```python
from build123d import *

# Parameters (mm, degrees)
BOSS_EXTRUDE1_DEPTH = 6.1
CUT_EXTRUDE1_DEPTH  = 1


with BuildPart() as part:
    # Sketch1 → Boss-Extrude1 (new body)
    with BuildSketch(Plane(origin=(0, 0, 0), x_dir=(1, 0, 0), z_dir=(0, 1, 0))):
        with BuildLine():
            ThreePointArc((-2.603734293, 13.735096717), (-4.043681259, 12.445171239), (-5.966821997, 12.642363282))
            Line((-5.966821997, 12.642363282), (-6.843279813, 13.183422247))
            Line((-6.843279813, 13.183422247), (-7.052164592, 13.353548445))
            Line((-7.052164592, 13.353548445), (-7.399861002, 13.637560961))
            Line((-7.399861002, 13.637560961), (-7.793732744, 13.973879308))
            Line((-7.793732744, 13.973879308), (-8.226942264, 14.264456075))
            Line((-8.226942264, 14.264456075), (-9.020650473, 14.599698524))
            Line((-9.020650473, 14.599698524), (-9.172029908, 14.639881345))
            Line((-9.172029908, 14.639881345), (-11.091125587, 13.245576719))
            Line((-11.091125587, 13.245576719), (-11.051137643, 12.366770586))
            Line((-11.051137643, 12.366770586), (-10.799290258, 11.512249619))
            Line((-10.799290258, 11.512249619), (-10.485832024, 10.75420757))
            Line((-10.485832024, 10.75420757), (-10.259959226, 9.993083115))
            Line((-10.259959226, 9.993083115), (-10.179752581, 9.581490045))
            ThreePointArc((-10.179752581, 9.581490045), (-10.586494975, 7.691538822), (-12.258255089, 6.720676771))
            Line((-12.258255089, 6.720676771), (-13.285350838, 6.643233691))
            Line((-13.285350838, 6.643233691), (-13.554339843, 6.658089283))
            Line((-13.554339843, 6.658089283), (-14.002570517, 6.683489414))
            Line((-14.002570517, 6.683489414), (-14.518902414, 6.72406467))
            Line((-14.518902414, 6.72406467), (-15.040173016, 6.704512046))
            Line((-15.040173016, 6.704512046), (-15.879347013, 6.509198904))
            Line((-15.879347013, 6.509198904), (-16.025434419, 6.452728891))
            Line((-16.025434419, 6.452728891), (-16.75846374, 4.196696614))
            Line((-16.75846374, 4.196696614), (-16.20956353, 3.509231842))
            Line((-16.20956353, 3.509231842), (-15.503539893, 2.965942036))
            Line((-15.503539893, 2.965942036), (-14.804380918, 2.536919263))
            Line((-14.804380918, 2.536919263), (-14.174268255, 2.053921344))
            Line((-14.174268255, 2.053921344), (-13.86745138, 1.768079839))
            ThreePointArc((-13.86745138, 1.768079839), (-13.085627432, 0), (-13.86745138, -1.768079839))
            Line((-13.86745138, -1.768079839), (-14.652869395, -2.434444341))
            Line((-14.652869395, -2.434444341), (-14.87921797, -2.580533684))
            Line((-14.87921797, -2.580533684), (-15.256774024, -2.823447927))
            Line((-15.256774024, -2.823447927), (-15.698344841, -3.094114129))
            Line((-15.698344841, -3.094114129), (-16.108568873, -3.416327706))
            Line((-16.108568873, -3.416327706), (-16.672672713, -4.067593457))
            Line((-16.672672713, -4.067593457), (-16.757667666, -4.19914668))
            Line((-16.757667666, -4.19914668), (-16.024638344, -6.455178957))
            Line((-16.024638344, -6.455178957), (-15.176487091, -6.688714191))
            Line((-15.176487091, -6.688714191), (-14.285964235, -6.713254596))
            Line((-14.285964235, -6.713254596), (-13.468159483, -6.649385976))
            Line((-13.468159483, -6.649385976), (-12.674488577, -6.66976857))
            Line((-12.674488577, -6.66976857), (-12.258255089, -6.720676771))
            ThreePointArc((-12.258255089, -6.720676771), (-10.586494975, -7.691538822), (-10.179752581, -9.581490045))
            Line((-10.179752581, -9.581490045), (-10.423489876, -10.582247377))
            Line((-10.423489876, -10.582247377), (-10.520740558, -10.833480493))
            Line((-10.520740558, -10.833480493), (-10.683408413, -11.251924125))
            Line((-10.683408413, -11.251924125), (-10.881553106, -11.730446496))
            Line((-10.881553106, -11.730446496), (-11.02403893, -12.232246392))
            Line((-11.02403893, -12.232246392), (-11.09760412, -13.09070337))
            Line((-11.09760412, -13.09070337), (-11.089041437, -13.247090943))
            Line((-11.089041437, -13.247090943), (-9.169945757, -14.641395569))
            Line((-9.169945757, -14.641395569), (-8.346508413, -14.331798745))
            Line((-8.346508413, -14.331798745), (-7.611635801, -13.828216148))
            Line((-7.611635801, -13.828216148), (-6.987558891, -13.295851776))
            Line((-6.987558891, -13.295851776), (-6.333485052, -12.845833588))
            Line((-6.333485052, -12.845833588), (-5.966821997, -12.642363282))
            ThreePointArc((-5.966821997, -12.642363282), (-4.043681259, -12.445171239), (-2.603734293, -13.735096717))
            Line((-2.603734293, -13.735096717), (-2.212691506, -14.687991594))
            Line((-2.212691506, -14.687991594), (-2.14369784, -14.94840597))
            Line((-2.14369784, -14.94840597), (-2.029343904, -15.382547746))
            Line((-2.029343904, -15.382547746), (-1.908377935, -15.886147005))
            Line((-1.908377935, -15.886147005), (-1.72870081, -16.375862714))
            Line((-1.72870081, -16.375862714), (-1.283627947, -17.113609532))
            Line((-1.283627947, -17.113609532), (-1.184778282, -17.235096718))
            Line((-1.184778282, -17.235096718), (1.187354434, -17.235096718))
            Line((1.187354434, -17.235096718), (1.671552791, -16.500623298))
            Line((1.671552791, -16.500623298), (1.970078799, -15.661269135))
            Line((1.970078799, -15.661269135), (2.162051698, -14.863754107))
            Line((2.162051698, -14.863754107), (2.426694495, -14.115226788))
            Line((2.426694495, -14.115226788), (2.603734293, -13.735096717))
            ThreePointArc((2.603734293, -13.735096717), (4.043681259, -12.445171239), (5.966821997, -12.642363282))
            Line((5.966821997, -12.642363282), (6.843279813, -13.183422247))
            Line((6.843279813, -13.183422247), (7.052164592, -13.353548445))
            Line((7.052164592, -13.353548445), (7.399861002, -13.637560961))
            Line((7.399861002, -13.637560961), (7.793732744, -13.973879308))
            Line((7.793732744, -13.973879308), (8.226942264, -14.264456075))
            Line((8.226942264, -14.264456075), (9.020650473, -14.599698524))
            Line((9.020650473, -14.599698524), (9.172029908, -14.639881345))
            Line((9.172029908, -14.639881345), (11.091125587, -13.245576719))
            Line((11.091125587, -13.245576719), (11.051137643, -12.366770586))
            Line((11.051137643, -12.366770586), (10.799290258, -11.512249619))
            Line((10.799290258, -11.512249619), (10.485832024, -10.75420757))
            Line((10.485832024, -10.75420757), (10.259959226, -9.993083115))
            Line((10.259959226, -9.993083115), (10.179752581, -9.581490045))
            ThreePointArc((10.179752581, -9.581490045), (10.586494975, -7.691538822), (12.258255089, -6.720676771))
            Line((12.258255089, -6.720676771), (13.285350838, -6.643233691))
            Line((13.285350838, -6.643233691), (13.554339843, -6.658089283))
            Line((13.554339843, -6.658089283), (14.002570517, -6.683489414))
            Line((14.002570517, -6.683489414), (14.518902414, -6.72406467))
            Line((14.518902414, -6.72406467), (15.040173016, -6.704512046))
            Line((15.040173016, -6.704512046), (15.879347013, -6.509198904))
            Line((15.879347013, -6.509198904), (16.025434419, -6.452728891))
            Line((16.025434419, -6.452728891), (16.75846374, -4.196696614))
            Line((16.75846374, -4.196696614), (16.20956353, -3.509231842))
            Line((16.20956353, -3.509231842), (15.503539893, -2.965942036))
            Line((15.503539893, -2.965942036), (14.804380918, -2.536919263))
            Line((14.804380918, -2.536919263), (14.174268255, -2.053921344))
            Line((14.174268255, -2.053921344), (13.86745138, -1.768079839))
            ThreePointArc((13.86745138, -1.768079839), (13.085627432, 0), (13.86745138, 1.768079839))
            Line((13.86745138, 1.768079839), (14.652869395, 2.434444341))
            Line((14.652869395, 2.434444341), (14.87921797, 2.580533684))
            Line((14.87921797, 2.580533684), (15.256774024, 2.823447927))
            Line((15.256774024, 2.823447927), (15.698344841, 3.094114129))
            Line((15.698344841, 3.094114129), (16.108568873, 3.416327706))
            Line((16.108568873, 3.416327706), (16.672672713, 4.067593457))
            Line((16.672672713, 4.067593457), (16.757667666, 4.19914668))
            Line((16.757667666, 4.19914668), (16.024638344, 6.455178957))
            Line((16.024638344, 6.455178957), (15.176487091, 6.688714191))
            Line((15.176487091, 6.688714191), (14.285964235, 6.713254596))
            Line((14.285964235, 6.713254596), (13.468159483, 6.649385976))
            Line((13.468159483, 6.649385976), (12.674488577, 6.66976857))
            Line((12.674488577, 6.66976857), (12.258255089, 6.720676771))
            ThreePointArc((12.258255089, 6.720676771), (10.586494975, 7.691538822), (10.179752581, 9.581490045))
            Line((10.179752581, 9.581490045), (10.423489876, 10.582247377))
            Line((10.423489876, 10.582247377), (10.520740558, 10.833480493))
            Line((10.520740558, 10.833480493), (10.683408413, 11.251924125))
            Line((10.683408413, 11.251924125), (10.881553106, 11.730446496))
            Line((10.881553106, 11.730446496), (11.02403893, 12.232246392))
            Line((11.02403893, 12.232246392), (11.09760412, 13.09070337))
            Line((11.09760412, 13.09070337), (11.089041437, 13.247090943))
            Line((11.089041437, 13.247090943), (9.169945757, 14.641395569))
            Line((9.169945757, 14.641395569), (8.346508413, 14.331798745))
            Line((8.346508413, 14.331798745), (7.611635801, 13.828216148))
            Line((7.611635801, 13.828216148), (6.987558891, 13.295851776))
            Line((6.987558891, 13.295851776), (6.333485052, 12.845833588))
            Line((6.333485052, 12.845833588), (5.966821997, 12.642363282))
            ThreePointArc((5.966821997, 12.642363282), (4.043681259, 12.445171239), (2.603734293, 13.735096717))
            Line((2.603734293, 13.735096717), (2.212691506, 14.687991594))
            Line((2.212691506, 14.687991594), (2.14369784, 14.94840597))
            Line((2.14369784, 14.94840597), (2.029343904, 15.382547746))
            Line((2.029343904, 15.382547746), (1.908377935, 15.886147005))
            Line((1.908377935, 15.886147005), (1.72870081, 16.375862714))
            Line((1.72870081, 16.375862714), (1.283627947, 17.113609532))
            Line((1.283627947, 17.113609532), (1.184778282, 17.235096718))
            Line((1.184778282, 17.235096718), (-1.187354434, 17.235096718))
            Line((-1.187354434, 17.235096718), (-1.671552791, 16.500623298))
            Line((-1.671552791, 16.500623298), (-1.970078799, 15.661269135))
            Line((-1.970078799, 15.661269135), (-2.162051698, 14.863754107))
            Line((-2.162051698, 14.863754107), (-2.426694495, 14.115226788))
            Line((-2.426694495, 14.115226788), (-2.603734293, 13.735096717))
        make_face()
    extrude(amount=BOSS_EXTRUDE1_DEPTH)

    # Sketch3 → Cut-Extrude1 (cut)
    with BuildSketch(Plane(origin=(0, 6.1, 0), x_dir=(1, 0, 0), z_dir=(0, 1, 0))):
        Polygon((-8.393092124, 4.285361852), (-8.393092124, -2.575657901), (-4.396381589, -2.575657901), (-4.396381589, -1.575657901), (-7.393092124, -1.575657901), (-7.393092124, 4.285361852), align=None)
    extrude(amount=-CUT_EXTRUDE1_DEPTH, mode=Mode.SUBTRACT)


solid = part.part
```
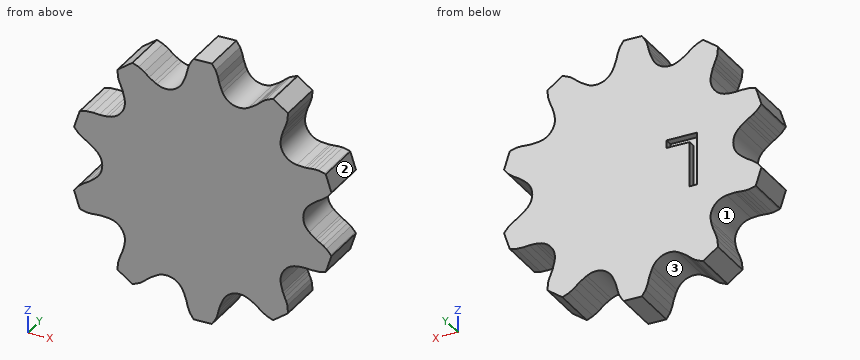
Can you work these out from the model? Positions are in its coordinate system, mm. Face numbers are marked on the shaded views. Coordinates: 2 decimals unless noted, no trailing zeros. Loops run counter-clockwise (first coordinate to the right, second up) from the corner with the lowest first, then second, coordinate; pieces in that order, holes last. Notation, with made-up numbers: (30, 14) -> (64, 14) arc R19 cw to (64, 20) -> close; hole circle Ø10 at (-31.75, 24). An arc over 180 degrees is marked (long way). Put each result on its own line as item: value. Start each with the question number.
Q1. I want a section at B-B (x = 5). Write out the boundary of the cut face in (y, z).
Q2. I want a section at A-A (z = -0.5). Write out the boundary of the cut face in (x, y).
Q3. Thinking about a two-plate mould opening in Z: for the marked faces 1, 2 and 3, which applies, pulls with the +Z half, pulls with the -Z half, needs draft (parallel to the pull), parting line crosses it, or undercut?
Q4. I'm going to push flat-ended pins straight in: P1, Ø2, axis at x = -13, y = 4, coming from the -Z side; P2, Ø0.8, axis at y = 5.5, z = 2, coming from the -X side; P3, Ø0.5, axis at x = -6.5, y = 6, coming from the +Z side. Where does each tip first touch, or does it pass through?
Q5. If I drill on line 1 (X direction, y = 2, z = 13); line 2 (Z direction, x = 1.5, y = 4.5); line 3 (Z direction, x = 13, y = 1.5), over which ranges is the centre line in solid material (lowest first)? Write a range as [from, to].
Q6. I want a section at C-C (z = -6). Write out the boundary of the cut face in (x, y).
Taken from the geometry:
1. outline: (0, -12.34) -> (6.1, -12.34) -> (6.1, 12.34) -> (0, 12.34) -> close
2. outline: (-13.14, 0) -> (13.14, 0) -> (13.14, 6.1) -> (-7.39, 6.1) -> (-7.39, 5.1) -> (-8.39, 5.1) -> (-8.39, 6.1) -> (-13.14, 6.1) -> close
3. face 1: undercut
3. face 2: pulls with the +Z half
3. face 3: pulls with the -Z half
4. P1: stops at z = -6.76
4. P2: stops at x = -14.61
4. P3: stops at z = 13.13
5. line 1: x = [-11.09, -6.56], [-3.12, 3.12], [6.55, 11.08]
5. line 2: z = [-16.75, 16.76]
5. line 3: z = [-6.66, 6.66]
6. outline: (-16.17, 0) -> (16.17, 0) -> (16.17, 6.1) -> (-16.17, 6.1) -> close
